Could you check a few things on this model? Use its own coordinates, in mm. Face numbers are marked on the shaded views. A direction names the side the tool comes from. Give positions to 0.01 mm unless a question says otherwise; leave off trailing zeros. Write each loop counter-clockwise with the first axis right and the second up, starting at its lowest first coordinate (ties: lowest second). Pieces come first, ordered by that corner, then holes. Notation, with made-up numbers: (-30, 7.25) -> (-2, 7.25) arc R22 ccw to (-2, 40.25) -> close; hole circle Ø7 at (-31.5, 20.25). An arc over 180 degrees is marked (long way). Write item = value, one per line. Start each with the question number.
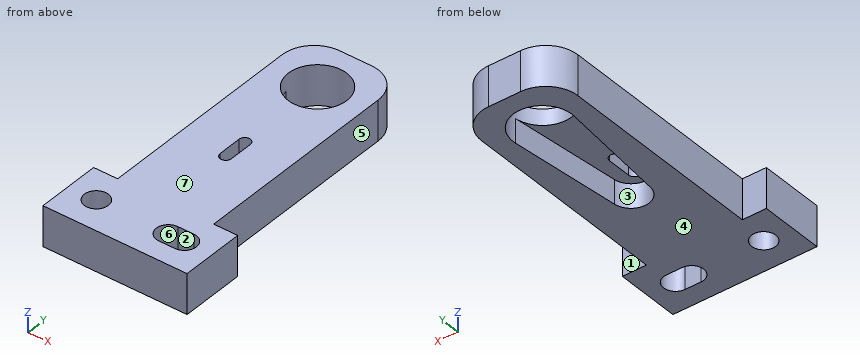
```python
from build123d import *

# Parameters (mm, degrees)
ESBO_O1_R                = 1.5
ESBO_O1_R_2              = 3.65
RESSALTO_EXTRUS_O1_DEPTH = 5
CORTE_EXTRUS_O1_DEPTH    = 3


with BuildPart() as part:
    # Esbo_o1 → Ressalto-extrus_o1 (new body)
    with BuildSketch(Plane.XY):
        with BuildLine():
            Line((-6, 2), (-6, -24))
            Line((-6, -24), (-9, -24))
            Line((-9, -24), (-9, -32))
            Line((-9, -32), (9, -32))
            Line((9, -32), (9, -24))
            Line((9, -24), (6, -24))
            Line((6, -24), (6, 2))
            ThreePointArc((6, 2), (4.828427125, 4.828427125), (2, 6))
            Line((2, 6), (-2, 6))
            ThreePointArc((-2, 6), (-4.828427125, 4.828427125), (-6, 2))
        make_face()
        with Locations((-5.5, -28)):
            Circle(ESBO_O1_R, mode=Mode.SUBTRACT)
        Circle(ESBO_O1_R_2, mode=Mode.SUBTRACT)
        with BuildLine():
            Line((-0.7, -14.5), (-0.7, -11.5))
            ThreePointArc((-0.7, -11.5), (0, -10.8), (0.7, -11.5))
            Line((0.7, -11.5), (0.7, -14.5))
            ThreePointArc((0.7, -14.5), (0, -15.2), (-0.7, -14.5))
        make_face(mode=Mode.SUBTRACT)
        with BuildLine():
            Line((5.5, -26.5), (3.5, -26.5))
            ThreePointArc((3.5, -26.5), (2, -28), (3.5, -29.5))
            Line((3.5, -29.5), (5.5, -29.5))
            ThreePointArc((5.5, -29.5), (7, -28), (5.5, -26.5))
        make_face(mode=Mode.SUBTRACT)
    extrude(amount=RESSALTO_EXTRUS_O1_DEPTH)

    # Esbo_o1_3 → Corte-extrus_o1 (cut)
    with BuildSketch(Plane.XY):
        with BuildLine():
            ThreePointArc((-2.238721733, -14.225), (0, -16.25), (2.238721733, -14.225))
            Line((2.238721733, -14.225), (3.631704145, -0.365))
            ThreePointArc((3.631704145, -0.365), (0, -3.65), (-3.631704145, -0.365))
            Line((-3.631704145, -0.365), (-2.238721733, -14.225))
        make_face()
        with BuildLine():
            ThreePointArc((0.7, -14.5), (0, -15.2), (-0.7, -14.5))
            Line((-0.7, -14.5), (-0.7, -11.5))
            ThreePointArc((-0.7, -11.5), (0, -10.8), (0.7, -11.5))
            Line((0.7, -11.5), (0.7, -14.5))
        make_face(mode=Mode.SUBTRACT)
    extrude(amount=CORTE_EXTRUS_O1_DEPTH, mode=Mode.SUBTRACT)


solid = part.part
```
(1) On a 3-axis mill with a long thin cutter (end or side, diameter ignored), from which of +Z, -Z, +X, -X, +Y, -Y can I reach the whole of each face in a straight line? I mean the marked faces 1, 2, 3 and 4. Say none if no direction works.
(2) We'd pull the mould along X, two halves only. Please class the marked faces 5, 6 and 7: released by +X, released by -X, zero draft, split by the parting line, or undercut.
(3) If I drill on line 1 along X through (y, z) = (-13.5, 3.2); line 2 along Y through (x, z) = (0, 1.35); line 3 along Z through (x, y) = (-1, -12.5), over which ranges is the centre line in solid material (lowest first)? Write a range as from..to.
(4) Imagine slicing it at C-C (z = 1.6). Please give me the cut outline in (x, y) (3 decimals), then the cut area to 3 significant figures.
(5) I'm going to push flat-ended pins straight in: pin 1 (2.5 mm diameter, centred on y = -7.5, z = 2, fed in from -X); pin 2 (1.5 mm diameter, centred on y = -5.5, z = 2.5, fed in from +X); pin 3 (0.9 mm diameter, centred on x = -8, z = 3, fed in from +Y). Where does each tip first touch, or does it pass through?
(6) Imagine slicing it at A-A (y = 0). Please give me the cut outline in (x, z).
(7) Imagine slicing it at B-B (x = 0). Please give me the cut outline in (y, z), then the cut area to 3 significant figures.
(8) Imagine slicing it at D-D (z = 4.15). Please give me the cut outline in (x, y).
Answers below:
q1.face_1 = +Z, -Z, +X, +Y
q1.face_2 = +Z, -Z
q1.face_3 = -Z
q1.face_4 = -Z, +X, -X, +Y, -Y
q2.face_5 = released by +X
q2.face_6 = undercut
q2.face_7 = zero draft
q3.line_1 = -6..-0.7, 0.7..6
q3.line_2 = -32..-16.25, 3.65..6
q3.line_3 = 3..5
q4.outline = (-9, -32) -> (9, -32) -> (9, -24) -> (6, -24) -> (6, 2) arc R4 ccw to (2, 6) -> (-2, 6) arc R4 ccw to (-6, 2) -> (-6, -24) -> (-9, -24) -> close; hole circle Ø3 at (-5.5, -28); hole (-3.632, -0.365) -> (-2.239, -14.225) arc R2.25 ccw to (2.239, -14.225) -> (3.632, -0.365) arc R3.65 ccw (long way) to start; hole (3.5, -29.5) -> (5.5, -29.5) arc R1.5 ccw to (5.5, -26.5) -> (3.5, -26.5) arc R1.5 ccw to start
q4.area = 365 mm^2
q5.pin_1 = -6
q5.pin_2 = 6
q5.pin_3 = -24
q6.outline = (-6, 0) -> (-3.65, 0) -> (-3.65, 5) -> (-6, 5) -> close; (3.65, 0) -> (6, 0) -> (6, 5) -> (3.65, 5) -> close
q7.outline = (-32, 0) -> (-16.25, 0) -> (-16.25, 3) -> (-15.2, 3) -> (-15.2, 5) -> (-32, 5) -> close; (-10.8, 3) -> (-3.65, 3) -> (-3.65, 5) -> (-10.8, 5) -> close; (3.65, 0) -> (6, 0) -> (6, 5) -> (3.65, 5) -> close
q7.area = 107 mm^2
q8.outline = (-9, -32) -> (9, -32) -> (9, -24) -> (6, -24) -> (6, 2) arc R4 ccw to (2, 6) -> (-2, 6) arc R4 ccw to (-6, 2) -> (-6, -24) -> (-9, -24) -> close; hole circle Ø3 at (-5.5, -28); hole circle Ø7.3 at (0, 0); hole (-0.7, -14.5) arc R0.7 ccw to (0.7, -14.5) -> (0.7, -11.5) arc R0.7 ccw to (-0.7, -11.5) -> close; hole (3.5, -29.5) -> (5.5, -29.5) arc R1.5 ccw to (5.5, -26.5) -> (3.5, -26.5) arc R1.5 ccw to start
